Could you check a few things on this model? Use its own coordinates, in mm. Face numbers are marked on the shaded views. Coordinates: 2 decimals unless noted, no trailing zeros. Loops run counter-clockwise (first coordinate to the right, second up) from the corner with the lowest first, then second, coordinate; pieces in that order, holes last.
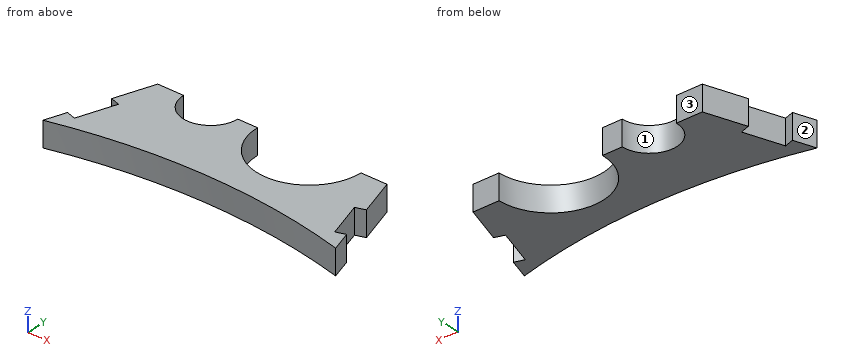
from build123d import *

# Parameters (mm, degrees)
BOSS_EXTRUDE2_DEPTH = 6.35


with BuildPart() as part:
    # Sketch1 → Boss-Extrude2 (new body)
    with BuildSketch(Plane.XY):
        with BuildLine():
            Line((37.717239544, 147.658964649), (35.965487423, 153.043027332))
            Line((35.965487423, 153.043027332), (33.550115758, 152.257164929))
            Line((33.550115758, 152.257164929), (30.406666146, 161.918651592))
            Line((30.406666146, 161.918651592), (32.822037812, 162.704513995))
            Line((32.822037812, 162.704513995), (29.545241798, 172.775844825))
            Line((29.545241798, 172.775844825), (22.8473, 172.775844825))
            ThreePointArc((22.8473, 172.775844825), (9.5123, 159.440844825), (-3.8227, 172.775844825))
            Line((-3.8227, 172.775844825), (-8.9027, 172.775844825))
            ThreePointArc((-8.9027, 172.775844825), (-15.8877, 165.790844825), (-22.8727, 172.775844825))
            Line((-22.8727, 172.775844825), (-29.545241798, 172.775844825))
            Line((-29.545241798, 172.775844825), (-32.822037812, 162.704513995))
            Line((-32.822037812, 162.704513995), (-30.406666146, 161.918651592))
            Line((-30.406666146, 161.918651592), (-33.550115758, 152.257164929))
            Line((-33.550115758, 152.257164929), (-35.965487423, 153.043027332))
            Line((-35.965487423, 153.043027332), (-37.717239544, 147.658964649))
            ThreePointArc((-37.717239544, 147.658964649), (0, 152.4), (37.717239544, 147.658964649))
        make_face()
    extrude(amount=BOSS_EXTRUDE2_DEPTH)


solid = part.part
(1) We'd pull the mould along X, two halves only. Please class the marked faces 1, 2 and 3: +X half, -X half, draft (parallel to the pull), parting line (faces both ways), or undercut.
Answers:
face 1: undercut
face 2: -X half
face 3: draft
(2) Imagine slicing it at C-C, the plane z = 1.5. Write out the boundary of the cut face in (x, y) (3 decimals).
Answers:
outline: (-37.717, 147.659) arc R152.4 cw to (37.717, 147.659) - (35.965, 153.043) - (33.55, 152.257) - (30.407, 161.919) - (32.822, 162.705) - (29.545, 172.776) - (22.847, 172.776) arc R13.335 cw to (-3.823, 172.776) - (-8.903, 172.776) arc R6.985 cw to (-22.873, 172.776) - (-29.545, 172.776) - (-32.822, 162.705) - (-30.407, 161.919) - (-33.55, 152.257) - (-35.965, 153.043) - close
(3) Imagine slicing it at B-B, the plane y = 166.75. Write out the boundary of the cut face in (x, z), and give its area (3 significant figures).
Answers:
outline: (-31.51, 0) - (-19.42, 0) - (-19.42, 6.35) - (-31.51, 6.35) - close; (-12.36, 0) - (-2.38, 0) - (-2.38, 6.35) - (-12.36, 6.35) - close; (21.41, 0) - (31.51, 0) - (31.51, 6.35) - (21.41, 6.35) - close
area: 204 mm2
(4) Imagine slicing it at A-A, the plane y = 151.5. Write out the boundary of the cut face in (x, z).
Answers:
outline: (-36.47, 0) - (-16.54, 0) - (-16.54, 6.35) - (-36.47, 6.35) - close; (16.54, 0) - (36.47, 0) - (36.47, 6.35) - (16.54, 6.35) - close
(5) Imagine slicing it at D-D, the plane x = -6. Write out the boundary of the cut face in (y, z).
Answers:
outline: (152.28, 0) - (172.78, 0) - (172.78, 6.35) - (152.28, 6.35) - close
(6) I need wall thicknesses on probe 1 along X at (y, z) = (166.75, 0.75); probe 2 along X at (y, z) = (161.5, 4.25); probe 3 along X at (y, z) = (163, 3.5). Which ranges of each line are inside material? Lowest first, please.
Answers:
probe 1: x = -31.51 to -19.42, -12.36 to -2.38, 21.41 to 31.51
probe 2: x = -30.54 to 2.39, 16.63 to 30.54
probe 3: x = -32.73 to 0.44, 18.58 to 32.73
(7) For pin 1 (1 mm diameter, centred on x = -26, z = 5, fed in from -Y); pin 2 (1 mm diameter, centred on x = -11.5, y = 162, fed in from -Z); pin 3 (1.5 mm diameter, centred on y = 170, z = 4, fed in from +X), each with a flat end and sliding along its axis, tell me the tip position at first contact or that it passes through.
Answers:
pin 1: stops at y = 150.08
pin 2: stops at z = 0
pin 3: stops at x = 30.69
